```python
from build123d import *

# Parameters (mm, degrees)
SKETCH1_W           = 20.6
SKETCH1_H           = 17
BOSS_EXTRUDE1_DEPTH = 7
SKETCH2_W           = 17.582410578
SKETCH2_H           = 4.15503942
BOSS_EXTRUDE2_DEPTH = 0.2
SKETCH3_W           = 0.284935897
SKETCH3_H           = 3.175
BOSS_EXTRUDE3_DEPTH = 0.2


with BuildPart() as part:
    # Sketch1 → Boss-Extrude1 (new body)
    with BuildSketch(Plane(origin=(0, 0, 0), x_dir=(1, 0, 0), z_dir=(0, 1, 0))):
        Rectangle(SKETCH1_W, SKETCH1_H)
    extrude(amount=BOSS_EXTRUDE1_DEPTH)

    # Sketch2 → Boss-Extrude2 (add)
    with BuildSketch(Plane.XY.offset(8.5)):
        with Locations((0, 3.5)):
            Rectangle(SKETCH2_W, SKETCH2_H)
    extrude(amount=BOSS_EXTRUDE2_DEPTH)

    # Sketch3 → Boss-Extrude3 (add)
    # profile 1 of 2: a face of its own
    with BuildSketch(Plane.XY.offset(8.7)):
        with Locations((-5.816789994, 3.509432337)):
            Rectangle(SKETCH3_W, SKETCH3_H)
    # profile 2 of 2: a face of its own
    with BuildSketch(Plane.XY.offset(8.7)):
        with BuildLine():
            add(Edge.make_bspline(
                [(5.173594622, 5.178342594), (5.232384832, 5.176853538), (5.347853656, 5.173928908), (5.517557313, 5.151541436), (5.679568578, 5.112810618), (5.835207204, 5.061227769), (5.982611547, 4.992417005), (6.122891114, 4.909245478), (6.255712135, 4.810841833), (6.379284388, 4.697966749), (6.492366051, 4.575154616), (6.591993819, 4.444092511), (6.675489328, 4.305572884), (6.744056435, 4.160011987), (6.797848745, 4.007739016), (6.834968163, 3.847942171), (6.8586792, 3.681656816), (6.861451226, 3.568239589), (6.862857443, 3.510704373)],
                knots=[0, 0, 0, 0, 1.065120563, 2.091984664, 3.0946048, 4.079830382, 5.057816894, 6.036188127, 7.030412546, 8.04752943, 9.064399622, 10.05169764, 11.02544977, 11.989514704, 12.962713494, 13.945757189, 14.957906945, 16, 16, 16, 16], degree=3))
            add(Edge.make_bspline(
                [(6.862857443, 3.510704373), (6.861451432, 3.453592975), (6.858680023, 3.341019794), (6.834941204, 3.175789669), (6.797711154, 3.016957394), (6.744555969, 2.864788124), (6.676315714, 2.719121334), (6.592264237, 2.580340311), (6.493257568, 2.448399559), (6.38058421, 2.324744499), (6.257756122, 2.211353936), (6.126011523, 2.112548956), (5.988313297, 2.027527786), (5.84288949, 1.95968831), (5.691668742, 1.905466639), (5.533297635, 1.868498182), (5.368518261, 1.844652079), (5.256149565, 1.841913853), (5.199035327, 1.840522081)],
                knots=[0, 0, 0, 0, 1.043624062, 2.057103931, 3.04512605, 4.022047818, 4.998200453, 5.980619268, 6.982898556, 8.009068085, 9.034988726, 10.034168286, 11.015286542, 11.987931943, 12.962482838, 13.94673481, 14.956375938, 16, 16, 16, 16], degree=3))
            add(Edge.make_bspline(
                [(5.199035327, 1.840522081), (5.141500409, 1.841927596), (5.028083771, 1.844698241), (4.86158946, 1.868448515), (4.701680364, 1.905588127), (4.548813774, 1.958664544), (4.402904445, 2.027260174), (4.263667012, 2.110902718), (4.131660357, 2.210150625), (4.007978916, 2.322787446), (3.894813572, 2.445407354), (3.796153281, 2.576792714), (3.712491928, 2.714365878), (3.64412662, 2.858508632), (3.590002431, 3.008524155), (3.553077346, 3.165413131), (3.529186876, 3.328281112), (3.526433836, 3.439172884), (3.52503693, 3.49543995)],
                knots=[0, 0, 0, 0, 1.053102029, 2.075944431, 3.073151272, 4.055350789, 5.033113405, 6.020478099, 7.024410459, 8.052272461, 9.079885166, 10.07527673, 11.055994387, 12.023226415, 12.992069828, 13.970394897, 14.97016774, 16, 16, 16, 16], degree=3))
            add(Edge.make_bspline(
                [(3.52503693, 3.49543995), (3.525521921, 3.533206728), (3.526485784, 3.60826384), (3.538089676, 3.719721399), (3.554927791, 3.829386495), (3.579059526, 3.936947284), (3.610620538, 4.042140463), (3.647860591, 4.145691512), (3.693344594, 4.246551033), (3.744762039, 4.345196824), (3.802149536, 4.440091139), (3.865536823, 4.529789046), (3.932697479, 4.615043236), (4.006324272, 4.693644447), (4.083990618, 4.767879264), (4.166956433, 4.836606871), (4.254715469, 4.900447005), (4.347645342, 4.957978315), (4.443456206, 5.010011244), (4.542222997, 5.054662494), (4.642604315, 5.092985707), (4.745070317, 5.124047027), (4.849348903, 5.148568946), (4.955667665, 5.165267045), (5.063941902, 5.176900534), (5.136886455, 5.177859839), (5.173594622, 5.178342594)],
                knots=[0, 0, 0, 0, 1.037015668, 2.060948919, 3.074880161, 4.083647147, 5.086022904, 6.090072063, 7.104153813, 8.122640571, 9.144368836, 10.147691507, 11.138137339, 12.123020368, 13.103399296, 14.087645067, 15.080126199, 16.082011238, 17.087798457, 18.072939717, 19.057185487, 20.037253025, 21.01195951, 21.997135196, 22.992090687, 24, 24, 24, 24], degree=3))
        make_face()
        with BuildLine():
            add(Edge.make_bspline(
                [(5.18758701, 4.852701568), (5.157456592, 4.852334275), (5.097483806, 4.8516032), (5.008325691, 4.841973229), (4.920340151, 4.828248258), (4.833509015, 4.808670736), (4.748195596, 4.78199706), (4.663604668, 4.751298521), (4.580507612, 4.713905103), (4.499178756, 4.671657007), (4.420334366, 4.624894772), (4.34593713, 4.573213241), (4.275794445, 4.517824409), (4.210078054, 4.458599014), (4.148980919, 4.395235447), (4.091300511, 4.328694308), (4.039348819, 4.257073664), (3.991736903, 4.182315652), (3.949130362, 4.104517646), (3.911243219, 4.0244987), (3.880251582, 3.941606084), (3.854976427, 3.856739098), (3.834021598, 3.770032153), (3.820746539, 3.68082749), (3.811010755, 3.589573352), (3.810321467, 3.527904099), (3.809972827, 3.496711985)],
                knots=[0, 0, 0, 0, 1.008559885, 2.007477868, 2.99961109, 3.989939068, 4.984837346, 5.991145699, 7.001802488, 8.033829008, 9.059044045, 10.069351652, 11.065060232, 12.050310815, 13.029377138, 14.011219647, 14.996725999, 15.989392538, 16.977580475, 17.965360261, 18.951710183, 19.937753436, 20.929683414, 21.935841486, 22.955955122, 24, 24, 24, 24], degree=3))
            add(Edge.make_bspline(
                [(3.809972827, 3.496711985), (3.811129309, 3.450844827), (3.813404467, 3.360609939), (3.83332312, 3.228377409), (3.864004482, 3.10129732), (3.909232236, 2.980065017), (3.965793151, 2.863638418), (4.035667544, 2.753050351), (4.118452572, 2.648270929), (4.212490199, 2.55003165), (4.315290083, 2.460364384), (4.42444906, 2.381657578), (4.538797689, 2.315063994), (4.658634166, 2.26081225), (4.783318719, 2.217822988), (4.913654784, 2.18836023), (5.048774129, 2.168969638), (5.140876938, 2.167107495), (5.18758701, 2.166163107)],
                knots=[0, 0, 0, 0, 1.032063989, 2.030389145, 3.003944642, 3.970395727, 4.937377036, 5.913328081, 6.909231446, 7.93887556, 8.970685674, 9.976071282, 10.964166581, 11.944589148, 12.933237628, 13.927779006, 14.949070134, 16, 16, 16, 16], degree=3))
            add(Edge.make_bspline(
                [(5.18758701, 2.166163107), (5.218982772, 2.166594457), (5.281249998, 2.167449954), (5.373865222, 2.176066611), (5.464811928, 2.189884093), (5.553962553, 2.20977833), (5.641215918, 2.234676868), (5.726936204, 2.264256735), (5.810210367, 2.301160398), (5.892088934, 2.341934612), (5.970462668, 2.388416755), (6.045279758, 2.438344219), (6.114654397, 2.493651468), (6.180321626, 2.551996912), (6.241669601, 2.614556974), (6.298283465, 2.681250318), (6.349972585, 2.752497914), (6.397566421, 2.827142532), (6.440023667, 2.905153419), (6.477016135, 2.985462484), (6.508399755, 3.067871976), (6.533734898, 3.152500758), (6.553588139, 3.2391881), (6.56726778, 3.328050071), (6.576836721, 3.418908903), (6.57755797, 3.480362258), (6.577921545, 3.51134039)],
                knots=[0, 0, 0, 0, 1.047197238, 2.076906641, 3.100256066, 4.114471768, 5.12198147, 6.126382909, 7.136867548, 8.15857795, 9.17633901, 10.174870724, 11.156907918, 12.133735059, 13.104061851, 14.077631395, 15.04955518, 16.038496417, 17.029181396, 18.010275684, 18.986308667, 19.968651475, 20.955262928, 21.950658345, 22.966943676, 24, 24, 24, 24], degree=3))
            add(Edge.make_bspline(
                [(6.577921545, 3.51134039), (6.577557678, 3.542106598), (6.576835882, 3.603137038), (6.567272351, 3.693362208), (6.553573686, 3.781584765), (6.533831801, 3.867458357), (6.508386304, 3.951004876), (6.477010655, 4.032145855), (6.440012562, 4.111183575), (6.397550815, 4.187922687), (6.349820747, 4.261559771), (6.297665255, 4.331956245), (6.240183832, 4.397790089), (6.179018795, 4.460686561), (6.112642349, 4.519304218), (6.041355168, 4.573662505), (5.966022689, 4.625073261), (5.886260125, 4.671451449), (5.803942396, 4.714281503), (5.719474734, 4.750976342), (5.633814051, 4.782156764), (5.547178177, 4.80875144), (5.458837904, 4.828171581), (5.369390145, 4.841985598), (5.278958653, 4.851599848), (5.218140875, 4.852333163), (5.18758701, 4.852701568)],
                knots=[0, 0, 0, 0, 1.02996197, 2.043119294, 3.035359645, 4.018872909, 4.991431989, 5.957985074, 6.929999688, 7.912076566, 8.892894881, 9.867085534, 10.843653904, 11.817741046, 12.803660682, 13.806313499, 14.818574707, 15.856120519, 16.894564902, 17.924820532, 18.937903209, 19.946497019, 20.957711757, 21.963978472, 22.977135795, 24, 24, 24, 24], degree=3))
        make_face(mode=Mode.SUBTRACT)
    extrude(amount=BOSS_EXTRUDE3_DEPTH)


solid = part.part
```
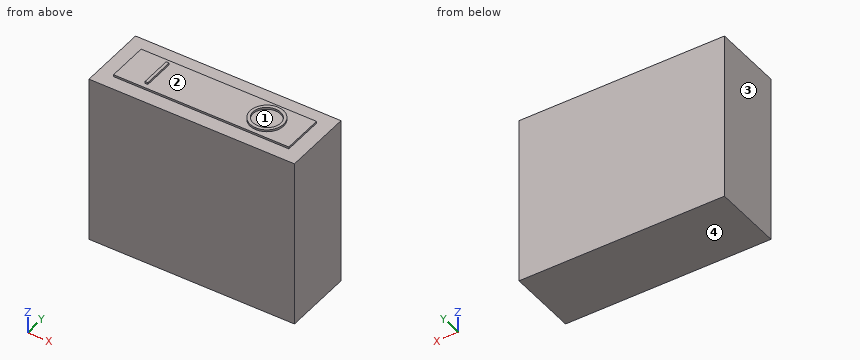
CAD build for the part. Positions are in the model's coordinates, mm. Face numbers are marked on the shaded views. Round coordinates to 2 decimals unless told otherwise and drop trailing zeros. Loops run counter-clockwise (first coordinate to the right, second up) from the corner with the lowest first, then second, coordinate; pieces in that order, holes last. Notation, with made-up numbers: M -1.5,55 L 2.5,55 A36 cw 2.5,90 Z; hole C 74,-9.5 d8. An arc over 180 degrees is marked long. Use a Markdown table: item, result. Add a question column.
(1) Cut at A-A (x = -4.5). Give the cut face in (y, z).
(2) Drill centre lines: line 1 (Z direction, x = 1.5, y = 5.75); line 2 (Z direction, x = -1.5, y = 4.75). Where is each one in solid material? Low to high.
(3) Flat gauge pins, fed straight in: pin 1 (3 mm diameter, centred on x = 5.5, y = 3, fed in from +Z); pin 2 (2 mm diameter, centred on x = -4.5, y = 3, fed in from +Z). Where does each tip first touch, or does it go through?
(4) Cut at B-B (y = 6). Give the cut face in (x, z).
(5) Pull direction X, two halves, no side cores. Call the marked faces 1, 2, 3 and 4: +X half, -X half, draft (parallel to the pull), parting line (faces both ways), or undercut.
Geometry says:
| question | item | result |
|---|---|---|
| 1 | outline | M 0,-8.5 L 7,-8.5 L 7,8.5 L 5.58,8.5 L 5.58,8.7 L 1.42,8.7 L 1.42,8.5 L 0,8.5 Z |
| 2 | line 1 | z = -8.5 to 8.5 |
| 2 | line 2 | z = -8.5 to 8.7 |
| 3 | pin 1 | stops at z = 8.9 |
| 3 | pin 2 | stops at z = 8.7 |
| 4 | outline | M -10.3,-8.5 L 10.3,-8.5 L 10.3,8.5 L -10.3,8.5 Z |
| 5 | face 1 | undercut |
| 5 | face 2 | undercut |
| 5 | face 3 | -X half |
| 5 | face 4 | draft |
